```python
from build123d import *

# Parameters (mm, degrees)
F0_W     = 110
F0_H     = 60
F1_DEPTH = 4
F3_DEPTH = 2


with BuildPart() as f1:
    # F0 (on Top) → F1 (new body)
    with BuildSketch(Plane.XY):
        with Locations((55, 30)):
            Rectangle(F0_W, F0_H)
    extrude(amount=F1_DEPTH)

    # F2 (on face) → F3 (join)
    with BuildSketch(Plane.XY.offset(4)):
        with BuildLine():
            ThreePointArc((7, 56), (6.12132, 53.87868), (4, 53))
            Line((4, 53), (2, 53))
            Line((2, 53), (2, 8))
            Line((2, 8), (4.5, 8))
            ThreePointArc((4.5, 8), (6.267767, 7.267767), (7, 5.5))
            Line((7, 5.5), (7, 2))
            Line((7, 2), (103, 2))
            Line((103, 2), (103, 4.5))
            ThreePointArc((103, 4.5), (103.732233, 6.267767), (105.5, 7))
            Line((105.5, 7), (108, 7))
            Line((108, 7), (108, 53))
            Line((108, 53), (105.5, 53))
            ThreePointArc((105.5, 53), (103.732233, 53.732233), (103, 55.5))
            Line((103, 55.5), (103, 58))
            Line((103, 58), (7, 58))
            Line((7, 58), (7, 56))
        make_face()
        with BuildLine():
            Line((4.5, 9.5), (3.5, 9.5))
            Line((3.5, 9.5), (3.5, 51.5))
            Line((3.5, 51.5), (4, 51.5))
            ThreePointArc((4, 51.5), (7.181981, 52.818019), (8.5, 56))
            Line((8.5, 56), (8.5, 56.5))
            Line((8.5, 56.5), (101.5, 56.5))
            Line((101.5, 56.5), (101.5, 55.5))
            ThreePointArc((101.5, 55.5), (102.671573, 52.671573), (105.5, 51.5))
            Line((105.5, 51.5), (106.5, 51.5))
            Line((106.5, 51.5), (106.5, 8.5))
            Line((106.5, 8.5), (105.5, 8.5))
            ThreePointArc((105.5, 8.5), (102.671573, 7.328427), (101.5, 4.5))
            Line((101.5, 4.5), (101.5, 3.5))
            Line((101.5, 3.5), (8.5, 3.5))
            Line((8.5, 3.5), (8.5, 5.5))
            ThreePointArc((8.5, 5.5), (7.328427, 8.328427), (4.5, 9.5))
        make_face(mode=Mode.SUBTRACT)
    extrude(amount=F3_DEPTH)


solid = f1.part
```
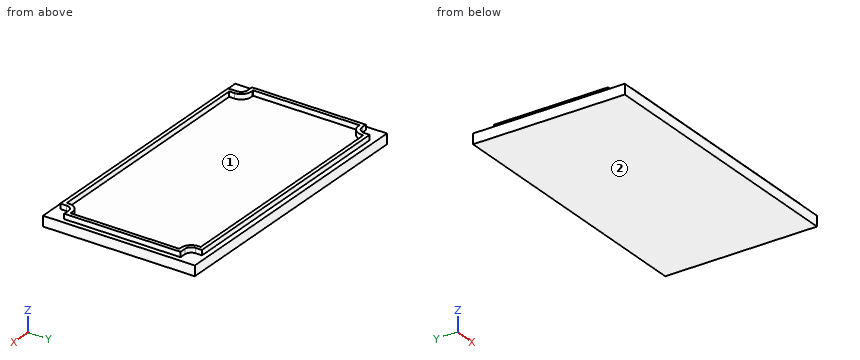
CAD build for the part. Positions are in the model's coordinates, mm. Face numbers are marked on the shaded views. Round coordinates to 2 decimals unless told otherwise and drop trailing zeros. Order: outer loops, then holes, each group sorted by start corner. A loop starts at its lowest first (then second) coordinate and runs counter-clockwise, first axis right, second up.
Q1. Two-plate mould, pull along Y, no slides. Class the marked faces 1 and 2: pulls with the +Y half, pulls with the -Y half, needs draft (parallel to the pull), parting line crosses it, or undercut.
Q2. Slice it at A-A (y = 50). Write the cut outline in (x, z), and give its area (3 significant figures).
Q3. Wall check: L1, parallel to X at y = 18.5, z = 4.6; L2, parallel to Y at x = 63, z = 4.35; L3, parallel to Z at x = 68, y = 42. Give the ranges that are in metal, low to high.
Q4. Slice it at B-B (x = 90). Write the cut outline in (y, z).
Q5. Drop flat-ended pins along their axis: pin 1 (2 mm diameter, centred on x = 63, y = 18.5, fed in from +Z); pin 2 (1 mm diameter, centred on y = 56.5, z = 5, fed in from +X); pin 3 (0.6 mm diameter, centred on x = 49.5, z = 5, fed in from +Y). Give the stop position or say it passes through.
Results below:
1. face 1: undercut
1. face 2: needs draft
2. outline: (0, 0) - (110, 0) - (110, 4) - (108, 4) - (108, 6) - (106.5, 6) - (106.5, 4) - (3.5, 4) - (3.5, 6) - (2, 6) - (2, 4) - (0, 4) - close
2. area: 446 mm2
3. L1: x = 2 to 3.5, 106.5 to 108
3. L2: y = 2 to 3.5, 56.5 to 58
3. L3: z = 0 to 4
4. outline: (0, 0) - (60, 0) - (60, 4) - (58, 4) - (58, 6) - (56.5, 6) - (56.5, 4) - (3.5, 4) - (3.5, 6) - (2, 6) - (2, 4) - (0, 4) - close
5. pin 1: stops at z = 4
5. pin 2: stops at x = 103
5. pin 3: stops at y = 58
